from build123d import *

# Parameters (mm, degrees)
SKETCH1_R           = 11.5
BOSS_EXTRUDE1_DEPTH = 5
SKETCH2_R           = 2.25
CUT_EXTRUDE1_DEPTH  = 18.014699527
CIRPATTERN1_COUNT   = 4
SKETCH3_R           = 9
BOSS_EXTRUDE2_DEPTH = 10
SKETCH4_R           = 2.1
CUT_EXTRUDE2_DEPTH  = 23.12464689
BOSS_EXTRUDE3_REACH = 30.627
SKETCH5_W           = 18
SKETCH5_H           = 10
SKETCH6_R           = 2.25
CUT_EXTRUDE3_DEPTH  = 10
CHAMFER2_SIZE       = 1
FILLET1_R           = 5
CUT_EXTRUDE4_DEPTH  = 20.091883144
SKETCH8_W           = 6
SKETCH8_H           = 3
CUT_EXTRUDE7_DEPTH  = 10
SKETCH9_W           = 3
SKETCH9_H           = 6
CUT_EXTRUDE8_DEPTH  = 6


with BuildPart() as part:
    # Sketch1 → Boss-Extrude1 (new body)
    with BuildSketch(Plane.XY):
        Circle(SKETCH1_R)
    extrude(amount=BOSS_EXTRUDE1_DEPTH)

    # Sketch2 → Cut-Extrude1 (cut, through all)
    with BuildSketch(Plane.XY.offset(5)):
        with Locations((0, 7)):
            Circle(SKETCH2_R)
    cut_extrude1 = extrude(amount=-CUT_EXTRUDE1_DEPTH, mode=Mode.SUBTRACT)

    # CirPattern1: Cut-Extrude1 ×4 about axis
    cirpattern1_axis = Axis((0, 0, 0), (0, 0, 1))
    for i in range(1, CIRPATTERN1_COUNT):
        add(cut_extrude1.rotate(cirpattern1_axis, i * 360 / CIRPATTERN1_COUNT), mode=Mode.SUBTRACT)

    # Sketch3 → Boss-Extrude2 (add)
    with BuildSketch(Plane.XY.offset(5)):
        with Locations(Location((0, 0, 0), (0, 0, 172.554009398))):
            Circle(SKETCH3_R)
    extrude(amount=BOSS_EXTRUDE2_DEPTH)

    # Sketch4 → Cut-Extrude2 (cut, through all)
    with BuildSketch(Plane.XY.offset(15)):
        Circle(SKETCH4_R)
    extrude(amount=-CUT_EXTRUDE2_DEPTH, mode=Mode.SUBTRACT)

    # Sketch5 → Boss-Extrude3 (add, up to next)
    with BuildSketch(Plane(origin=(0, 10, 0), x_dir=(1, 0, 0), z_dir=(0, 1, 0)), mode=Mode.PRIVATE) as boss_extrude3_sk1:
        with Locations((0, -10)):
            Rectangle(SKETCH5_W, SKETCH5_H)
    boss_extrude3_tool1 = extrude(boss_extrude3_sk1.sketch, amount=-BOSS_EXTRUDE3_REACH, mode=Mode.PRIVATE) - part.part
    add(boss_extrude3_tool1.solids().sort_by_distance((0, 10, 10))[0])

    # Sketch6 → Cut-Extrude3 (cut)
    with BuildSketch(Plane(origin=(0, 10, 0), x_dir=(1, 0, 0), z_dir=(0, 1, 0))):
        with Locations(Location((0, -10, 0), (0, 0, 270))):
            Circle(SKETCH6_R)
    extrude(amount=-CUT_EXTRUDE3_DEPTH, mode=Mode.SUBTRACT)

    # Chamfer2
    chamfer2_edges = [part.edges().sort_by_distance(p)[0] for p in [
        (-7, -2.25, 0),
        (2.25, -7, 0),
        (7, 2.25, 0),
        (-2.25, 7, 0),
    ]]
    chamfer(chamfer2_edges, length=CHAMFER2_SIZE)

    # Fillet1
    # the kernel refuses this fillet: 5 mm, written as the material it takes off along each edge
    with BuildSketch(Plane(origin=(-9, 10, 27.5), x_dir=(0, -1, 0), z_dir=(0, 0, -1)), Plane(origin=(9, 10, 5), x_dir=(0, -1, 0), z_dir=(0, 0, 1))) as fillet1_piece_1:
        with BuildLine():
            CenterArc((FILLET1_R, -FILLET1_R), FILLET1_R, 90, 90)
            Line((0, -FILLET1_R), (0, 0))
            Line((0, 0), (FILLET1_R, 0))
        make_face()
    extrude(amount=22.5, mode=Mode.SUBTRACT)

    # Sketch7 → Cut-Extrude4 (cut, through all)
    with BuildSketch(Plane(origin=(0, 0, 5), x_dir=(-1, 0, 0), z_dir=(0, 0, -1))):
        with BuildLine():
            Line((-9, 1.030776406), (-9, 0))
            ThreePointArc((-9, 0), (-8.981006744, -0.584395292), (-8.924107143, -1.166324013))
            ThreePointArc((-8.924107143, -1.166324013), (-4.751341115, 0.077673804), (-9, 1.030776406))
        make_face()
        with BuildLine():
            Line((9, 0), (9, 1.030776406))
            ThreePointArc((9, 1.030776406), (4.751341115, 0.077673804), (8.924107143, -1.166324013))
            ThreePointArc((8.924107143, -1.166324013), (8.981006744, -0.584395292), (9, 0))
        make_face()
    extrude(amount=-CUT_EXTRUDE4_DEPTH, mode=Mode.SUBTRACT)

    # Sketch8 → Cut-Extrude7 (cut)
    with BuildSketch(Plane.XY.offset(15)):
        with Locations((0, 4)):
            Rectangle(SKETCH8_W, SKETCH8_H)
    extrude(amount=-CUT_EXTRUDE7_DEPTH, mode=Mode.SUBTRACT)

    # Sketch9 → Cut-Extrude8 (cut)
    with BuildSketch(Plane(origin=(9, 0, 0), x_dir=(0, 0, -1), z_dir=(1, 0, 0))):
        with Locations((-6.5, 0)):
            Rectangle(SKETCH9_W, SKETCH9_H)
    cut_extrude8 = extrude(amount=-CUT_EXTRUDE8_DEPTH, mode=Mode.SUBTRACT)

    # Mirror1: Cut-Extrude8 across plane
    add(cut_extrude8.mirror(Plane(origin=(0, 0, 0), x_dir=(0, 0, 1), z_dir=(1, 0, 0))), mode=Mode.SUBTRACT)


solid = part.part
Geometry check sheet. Reference: the model listing, model coordinates, mm. A direction names the side the tool comes from. Give positions to 0.01 mm unless a question says otherwise; leave off trailing zeros. Loops run counter-clockwise (first coordinate to the right, second up) from the corner with the lowest first, then second, coordinate; pieces in that order, holes last. Notation, with made-up numbers: M -9.5,28 L -0.5,28 A12 ccw -0.5,45 Z; hole C -17,12.5 d6. An arc over 180 degrees is marked long. Write each question's results on one line, items separated by ' | '.
1) Section check A-A, the plane z = 6.5. Record the boundary of the cut face in (x, y).
Answers follow:
outline: M -9,3 L -3,3 L -3,5.5 L 3,5.5 L 3,3 L 9,3 L 9,5 A5 ccw 4,10 L -4,10 A5 ccw -9,5 Z; M -8.49,-3 A9 ccw 8.49,-3 L 3,-3 L 3,2.5 L -3,2.5 L -3,-3 Z; hole C 0,0 d4.2
2) Tool access check on faces 1 (the face through (1.21, 8.897, 3.028)), 2 (the face through (-0.9, 10, 7.7)), 3 (the face through (6, 3, 7)), 4 (the face through (-3, 4, 10)), 5 (the face through (-3, 0, 7)). Record the directions out of +Z, -Z, +X, -X, +Y, -Y that give a thin tool (end or side, any length) a straight path to the whole face; none if there is none.
Answers follow:
face 1: -Z | face 2: +Z, +X, -X, +Y | face 3: +X, -X | face 4: +Z | face 5: -X
3) Section check C-C, the plane z = 10. Record the boundary of the cut face in (x, y).
Answers follow:
outline: M -9,1.03 A2.25 cw long -8.92,-1.17 A9 ccw 8.92,-1.17 A2.25 cw long 9,1.03 L 9,5 A5 ccw 4,10 L 2.25,10 L 2.25,5.5 L 3,5.5 L 3,2.5 L 2.25,2.5 L 2.25,0 L 2.1,0 A2.1 cw -2.1,0 L -2.25,0 L -2.25,2.5 L -3,2.5 L -3,5.5 L -2.25,5.5 L -2.25,10 L -4,10 A5 ccw -9,5 Z
4) Release check for a two-part mould opening along X. For faces 6 (the face through (9, 3, 11)), 7 (the face through (-8.897, 1.21, 3.028)), 8 (the face through (4.7, -0.7, 8)) record: +X half, -X half, draft (parallel to the pull), parting line (faces both ways), or undercut.
Answers follow:
face 6: +X half | face 7: undercut | face 8: draft
5) Thickness scan on line 1 (Y direction, x = 0, z = 3.3); line 2 (X direction, y = 5.25, z = 12.5); line 3 (Y direction, x = -7, z = 3.1). Record the ranges inside material, lowest first.
Answers follow:
line 1: -11.5 to -9.25, -4.75 to -2.1, 2.1 to 4.75, 9.25 to 11.5 | line 2: -8.99 to -3, 3 to 8.99 | line 3: -9.12 to -2.25, 2.25 to 9.12
6) Section check D-D, the plane y = 7. Record the boundary of the cut face in (x, z).
Answers follow:
outline: M -9.12,0 L -3.25,0 L -2.25,1 L -2.25,5 L 2.25,5 L 2.25,1 L 3.25,0 L 9.12,0 L 9.12,5 L 8.58,5 L 8.58,15 L -8.58,15 L -8.58,5 L -9.12,5 Z; hole C 0,10 d4.5
7) Gauge pin test, flat ends, axial feed: pin 1 (0.9 mm diameter, centred on y = 1, z = 6, fed in from +X); pin 2 (2.5 mm diameter, centred on x = -7, y = 0, fed in from -Z); pin 3 (2.5 mm diameter, centred on y = -1.5, z = 6.5, fed in from -X); pin 4 (0.9 mm diameter, centred on x = 6, z = 6, fed in from -Y) (3 decimals). Record the tip position at first contact, or that the pin passes through.
Answers follow:
pin 1: x = 3 | pin 2: through | pin 3: x = -3 | pin 4: y = -7.085
8) Section check B-B, the plane x = -7. Record the boundary of the cut face in (y, z), plus the area to 3 significant figures.
Answers follow:
outline: M -9.12,0 L -3.25,0 L -2.25,1 L -2.25,5 L -3,5 L -3,8 L -2.25,8 L -2.25,15 L -5.66,15 L -5.66,5 L -9.12,5 Z; M 2.25,1 L 3.25,0 L 9.12,0 L 9.12,5 L 9,5 L 9,15 L 2.25,15 L 2.25,8 L 3,8 L 3,5 L 2.25,5 Z | area: 165 mm2
